from build123d import *

# Parameters (mm, degrees)
SKETCH1_W                    = 60
SKETCH1_H                    = 80
BASE_FLANGE1_DEPTH           = 3
EDGE_FLANGE1_START           = -30
EDGE_FLANGE1_DEPTH           = 60
EDGE_FLANGE1_2_DEPTH         = 60
EDGE_FLANGE2_STRIP_W         = 14
EDGE_FLANGE2_STRIP_H         = 3
EDGE_FLANGE2_STRIP_CUT_DEPTH = 60
EDGE_FLANGE2_DEPTH           = 60
EDGE_FLANGE3_STRIP_W         = 14
EDGE_FLANGE3_STRIP_H         = 3
EDGE_FLANGE3_STRIP_CUT_DEPTH = 60
EDGE_FLANGE3_DEPTH           = 60
SKETCH17_R                   = 4.2
CUT_EXTRUDE1_DEPTH           = 10
SKETCH18_R                   = 4.2
CUT_EXTRUDE2_DEPTH           = 10


# Read off the part's stored shape, not the designer's step: Edge-Flange1
# Sheet-metal steps are written as plain solids
with BuildPart() as part:
    # Sketch1 → Base-Flange1 (new body)
    with BuildSketch(Plane.XY):
        Rectangle(SKETCH1_W, SKETCH1_H)
    extrude(amount=-BASE_FLANGE1_DEPTH)

    # Edge-Flange1 outline → Edge-Flange1 (cut)
    with BuildSketch(Plane.YZ.offset(EDGE_FLANGE1_START)):
        with BuildLine():
            ThreePointArc((35.343145751, 0), (36.87387948, -0.30448187), (38.171572875, -1.171572875))
            Line((38.171572875, -1.171572875), (40, -3))
            Line((40, -3), (40, 0))
            Line((40, 0), (35.343145751, 0))
        make_face()
    extrude(amount=EDGE_FLANGE1_DEPTH, mode=Mode.SUBTRACT)

    # Edge-Flange1 2 outline → Edge-Flange1 2 (add)
    with BuildSketch(Plane.YZ.offset(EDGE_FLANGE1_START)):
        with BuildLine():
            Line((107.710678119, -70.710678119), (40, -3))
            Line((40, -3), (35.343145751, -3))
            ThreePointArc((35.343145751, -3), (35.725829183, -3.076120467), (36.050252532, -3.292893219))
            Line((36.050252532, -3.292893219), (105.589357775, -72.831998462))
            Line((105.589357775, -72.831998462), (107.710678119, -70.710678119))
        make_face()
    extrude(amount=EDGE_FLANGE1_2_DEPTH)

    # Edge-Flange2 strip (across the edge) → Edge-Flange2 strip cut (cut)
    with BuildSketch(Plane(origin=(30, -40, -3), x_dir=(0, 1, 0), z_dir=(-1, 0, 0))):
        with Locations((-3, -1.5)):
            Rectangle(EDGE_FLANGE2_STRIP_W, EDGE_FLANGE2_STRIP_H)
    extrude(amount=EDGE_FLANGE2_STRIP_CUT_DEPTH, mode=Mode.SUBTRACT)

    # Edge-Flange2 section (across the edge) → Edge-Flange2 (add)
    with BuildSketch(Plane(origin=(30, -40, -3), x_dir=(0, 1, 0), z_dir=(-1, 0, 0))):
        with BuildLine():
            Line((0, 1), (0, 47))
            Line((0, 47), (3, 47))
            Line((3, 47), (3, 1))
            ThreePointArc((3, 1), (3.292893219, 0.292893219), (4, 0))
            Line((4, 0), (4, -3))
            ThreePointArc((4, -3), (1.171572875, -1.828427125), (0, 1))
        make_face()
    extrude(amount=EDGE_FLANGE2_DEPTH)

    # Edge-Flange3 strip (across the edge) → Edge-Flange3 strip cut (cut)
    with BuildSketch(Plane(origin=(30, -37, -50), x_dir=(0, 0, 1), z_dir=(-1, 0, 0))):
        with Locations((-3, -1.5)):
            Rectangle(EDGE_FLANGE3_STRIP_W, EDGE_FLANGE3_STRIP_H)
    extrude(amount=EDGE_FLANGE3_STRIP_CUT_DEPTH, mode=Mode.SUBTRACT)

    # Edge-Flange3 section (across the edge) → Edge-Flange3 (add)
    with BuildSketch(Plane(origin=(30, -37, -50), x_dir=(0, 0, 1), z_dir=(-1, 0, 0))):
        with BuildLine():
            Line((0, 1), (0, 12))
            Line((0, 12), (3, 12))
            Line((3, 12), (3, 1))
            ThreePointArc((3, 1), (3.292893219, 0.292893219), (4, 0))
            Line((4, 0), (4, -3))
            ThreePointArc((4, -3), (1.171572875, -1.828427125), (0, 1))
        make_face()
    extrude(amount=EDGE_FLANGE3_DEPTH)

    # Sketch17 → Cut-Extrude1 (cut)
    with BuildSketch(Plane.XZ.offset(40)):
        with Locations(Location((0, -25, 0), (0, 0, 270))):
            Circle(SKETCH17_R)
    extrude(amount=-CUT_EXTRUDE1_DEPTH, mode=Mode.SUBTRACT)

    # Sketch18 → Cut-Extrude2 (cut)
    with BuildSketch(Plane(origin=(0, 18.5, 18.5), x_dir=(1, 0, 0), z_dir=(0, 0.7071067811865438, 0.7071067811865513))):
        with Locations(Location((-18, 101.162950904, 0), (0, 0, 270))):
            Circle(SKETCH18_R)
        with Locations(Location((18, 101.162950904, 0), (0, 0, 270))):
            Circle(SKETCH18_R)
        with Locations(Location((18, 51.162950904, 0), (0, 0, 270))):
            Circle(SKETCH18_R)
        with Locations(Location((-18, 51.162950904, 0), (0, 0, 270))):
            Circle(SKETCH18_R)
    extrude(amount=-CUT_EXTRUDE2_DEPTH, mode=Mode.SUBTRACT)


solid = part.part
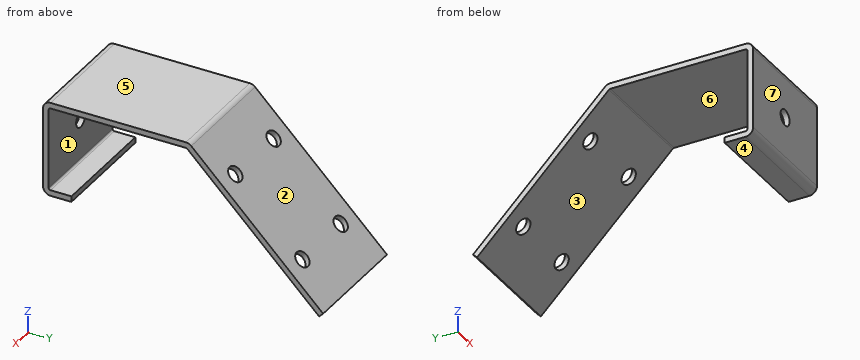
Source: CAD feature listing. Evaluate the final solid. Frame: model axes, mm. Face numbers are marked on the shaded views. A direction names the side the tool comes from. Coordinates: 2 decimals unless noted, no trailing zeros. Loops run counter-clockwise (first coordinate to the right, second up) from the corner with the lowest first, then second, coordinate; pieces in that order, holes last. Notation, with made-up numbers: (17, -21) - (40, -21) arc R37 cw to (40, 18) - close; hole circle Ø8 at (-40, 56.25). An arc over 180 degrees is marked (long way). One line per item, written item: value. Start each with the question number.
1. Set-up query: the marked faces 1, 2, 3 and 4. Return all of +Z, -Z, +X, -X, +Y, -Y with unobstructed straight access to the full face (end or side cutting, diameter ignored); none if empty.
2. Section C-C (x = 26.5). Return the cut outline in (y, z).
3. Mould query, pull axis Y, two halves, no side actions, for the marked faces 5, 6 and 7. Classes: pulls with the +Y half, pulls with the -Y half, needs draft (parallel to the pull), parting line crosses it, or undercut.
4. Ray query, L1, parallel to X at y = -38.8, z = -25; L2, parallel to Z at x = 6, y = 1.5; L3, parallel to Y at x = -12, z = -11. Return the intervals inside material, ascending.
5. Section A-A (x = 0). Return the cut outline in (y, z), and give its area (3 significant figures).
6. Section B-B (z = -25). Return the cut outline in (x, y), and give its area (3 significant figures).
7. Section D-D (z = -11). Return the cut outline in (x, y), and give its area (3 significant figures).
8. Contact query for flat-ended pins moving along their axis: P1, Ø9.5, axis at x = 0, z = -25, coming from the +Y side; P2, Ø6, axis at x = -10, y = 62, coming from the +Z side; P3, Ø4, axis at y = 55, z = -14, coming from the +X side; P4, Ø4, axis at x = -22.5, z = -16, coming from the +Y side. Output: stop coordinate, or through.
Verdict:
1. face 1: +X, -X
1. face 2: +Z, +X, -X, +Y
1. face 3: -Z, +X, -X
1. face 4: -Z, +X, -X, -Y
2. outline: (-40, -46) arc R4 ccw to (-36, -50) - (-25, -50) - (-25, -47) - (-36, -47) arc R1 cw to (-37, -46) - (-37, -4) arc R1 cw to (-36, -3) - (35.34, -3) arc R1 cw to (36.05, -3.29) - (105.59, -72.83) - (107.71, -70.71) - (38.17, -1.17) arc R4 ccw to (35.34, 0) - (-36, 0) arc R4 ccw to (-40, -4) - close
3. face 5: needs draft
3. face 6: undercut
3. face 7: pulls with the -Y half
4. L1: x = -30 to -4.2, 4.2 to 30
4. L2: z = -3 to 0
4. L3: y = -40 to -37, 43.76 to 48
5. outline: (-40, -46) arc R4 ccw to (-36, -50) - (-25, -50) - (-25, -47) - (-36, -47) arc R1 cw to (-37, -46) - (-37, -29.2) - (-40, -29.2) - close; (-40, -20.8) - (-37, -20.8) - (-37, -4) arc R1 cw to (-36, -3) - (35.34, -3) arc R1 cw to (36.05, -3.29) - (105.59, -72.83) - (107.71, -70.71) - (38.17, -1.17) arc R4 ccw to (35.34, 0) - (-36, 0) arc R4 ccw to (-40, -4) - close
5. area: 672 mm2
6. outline: (-30, -40) - (-4.2, -40) - (-4.2, -37) - (-30, -37) - close; (-30, 57.76) - (30, 57.76) - (30, 62) - (-30, 62) - close; (4.2, -40) - (30, -40) - (30, -37) - (4.2, -37) - close
6. area: 409 mm2
7. outline: (-30, -40) - (30, -40) - (30, -37) - (-30, -37) - close; (-30, 43.76) - (30, 43.76) - (30, 48) - (-30, 48) - close
7. area: 435 mm2
8. P1: stops at y = 66.75
8. P2: stops at z = -22
8. P3: passes through
8. P4: stops at y = 55
